For this review, take the finished solid that the model builds, in its own axes (mm). A direction names the side the tool comes from. Give positions to 0.01 mm unless a question says otherwise; leave off trailing zeros. Loops run counter-clockwise (first coordinate to the right, second up) from the corner with the lowest first, then second, coordinate; pieces in that order, holes last. Notation, with made-up numbers: (81.25, 73.25) - (140.25, 73.25) arc R14 cw to (140.25, 85.25) - close; hole circle Ø5 at (-27, -32). An arc over 180 degrees is marked (long way). Answer in a Markdown table with one row per item.
```python
from build123d import *

# Parameters (mm, degrees)
SKETCH_1_R          = 15.5
SKETCH_1_R_2        = 2
EXTRUDE_1_DEPTH     = 3
FILLET_1_R          = 3
SKETCH_5_R          = 15.5
SKETCH_5_R_2        = 2
EXTRUDE_3_DEPTH     = 2
EXTRUDE_5_DEPTH     = 7
FILLET_4_R          = 1
SKETCH_8_R          = 1.5
CUT_EXTRUDE_3_DEPTH = 35.179672449


with BuildPart() as part:
    # 草图1 → 凸台-拉伸1 (new body)
    with BuildSketch(Plane.XY):
        Circle(SKETCH_1_R)
        with Locations((-10.392304845, -6)):
            Circle(SKETCH_1_R_2, mode=Mode.SUBTRACT)
        with Locations((10.392304845, -6)):
            Circle(SKETCH_1_R_2, mode=Mode.SUBTRACT)
        with Locations((-10.392304845, 6)):
            Circle(SKETCH_1_R_2, mode=Mode.SUBTRACT)
        with BuildLine():
            ThreePointArc((2.604308084, 8.091203829), (5.825, 10.089195954), (5.705034021, 6.300998875))
            ThreePointArc((5.705034021, 6.300998875), (8.5, 0), (5.705034021, -6.300998875))
            ThreePointArc((5.705034021, -6.300998875), (5.825, -10.089195954), (2.604308084, -8.091203829))
            ThreePointArc((2.604308084, -8.091203829), (-4.25, -7.361215932), (-8.309342105, -1.790204954))
            ThreePointArc((-8.309342105, -1.790204954), (-11.65, 0), (-8.309342105, 1.790204954))
            ThreePointArc((-8.309342105, 1.790204954), (-4.25, 7.361215932), (2.604308084, 8.091203829))
        make_face(mode=Mode.SUBTRACT)
        with Locations((10.392304845, 6)):
            Circle(SKETCH_1_R_2, mode=Mode.SUBTRACT)
    extrude(amount=EXTRUDE_1_DEPTH)

    # 圆角1
    fillet_1_edges = [part.edges().sort_by_distance(p)[0] for p in [
        (-8.309342105, 1.790204954, 1.5),
        (-8.309342105, -1.790204954, 1.5),
        (2.604308084, -8.091203829, 1.5),
        (5.705034021, -6.300998875, 1.5),
        (5.705034021, 6.300998875, 1.5),
        (2.604308084, 8.091203829, 1.5),
    ]]
    fillet(fillet_1_edges, radius=FILLET_1_R)

    # 草图5 → 凸台-拉伸3 (add)
    with BuildSketch(Plane.XY.offset(3)):
        Circle(SKETCH_5_R)
        with Locations((-10.392304845, -6)):
            Circle(SKETCH_5_R_2, mode=Mode.SUBTRACT)
        with Locations((10.392304845, -6)):
            Circle(SKETCH_5_R_2, mode=Mode.SUBTRACT)
        with Locations((10.392304845, 6)):
            Circle(SKETCH_5_R_2, mode=Mode.SUBTRACT)
        with Locations((-10.392304845, 6)):
            Circle(SKETCH_5_R_2, mode=Mode.SUBTRACT)
    extrude(amount=EXTRUDE_3_DEPTH)

    # 草图7 → 凸台-拉伸5 (add)
    with BuildSketch(Plane.XY.offset(5)):
        with BuildLine():
            Line((9, 12.5), (-9, 12.5))
            Line((-9, 12.5), (-9, 9.481951639))
            ThreePointArc((-9, 9.481951639), (-7.287176573, 8.102540942), (-6.642304845, 6))
            ThreePointArc((-6.642304845, 6), (-7.287176573, 3.897459058), (-9, 2.518048361))
            Line((-9, 2.518048361), (-9, -2.518048361))
            ThreePointArc((-9, -2.518048361), (-7.287176573, -3.897459058), (-6.642304845, -6))
            ThreePointArc((-6.642304845, -6), (-7.287176573, -8.102540942), (-9, -9.481951639))
            Line((-9, -9.481951639), (-9, -12.5))
            Line((-9, -12.5), (9, -12.5))
            Line((9, -12.5), (9, -9.481951639))
            ThreePointArc((9, -9.481951639), (6.642304845, -6), (9, -2.518048361))
            Line((9, -2.518048361), (9, 2.518048361))
            ThreePointArc((9, 2.518048361), (6.642304845, 6), (9, 9.481951639))
            Line((9, 9.481951639), (9, 12.5))
        make_face()
    extrude(amount=EXTRUDE_5_DEPTH)

    # 圆角4
    fillet_4_edges = [part.edges().sort_by_distance(p)[0] for p in [
        (9, -9.481951639, 8.5),
        (9, -2.518048361, 8.5),
        (9, 2.518048361, 8.5),
        (9, 9.481951639, 8.5),
        (9, 12.5, 8.5),
        (-9, 12.5, 8.5),
        (-9, 9.481951639, 8.5),
        (-9, 2.518048361, 8.5),
        (-9, -2.518048361, 8.5),
        (-9, -9.481951639, 8.5),
        (-9, -12.5, 8.5),
        (9, -12.5, 8.5),
    ]]
    fillet(fillet_4_edges, radius=FILLET_4_R)

    # 草图8 → 切除-拉伸3 (cut, through all)
    with BuildSketch(Plane(origin=(0, 12.5, 0), x_dir=(1, 0, 0), z_dir=(0, 1, 0))):
        with Locations(Location((-4.75, -8.5, 0), (0, 0, 270))):
            Circle(SKETCH_8_R)
        with Locations(Location((4.75, -8.5, 0), (0, 0, 270))):
            Circle(SKETCH_8_R)
    extrude(amount=-CUT_EXTRUDE_3_DEPTH, mode=Mode.SUBTRACT)


solid = part.part
```
1. We need section A-A, the plane z = 8.5. Count the separate pieces of the cut face and the enclosed holes in it, and give its area (3 significant figures).
Values:
| item | result |
|---|---|
| separate pieces | 3 |
| enclosed holes | 0 |
| area | 251 mm^2 |
2. Clearance check with flat-ended pins moving along their axes: pin 1 (5.5 mm diameter, centred on x = 0, z = 8.5, fed in from -Y); pin 2 (5 mm diameter, centred on y = -7.5, z = 4, fed in from -X); pin 3 (2 mm diameter, centred on x = -3.5, z = 9.5, fed in from +Y). State where each tip first meets the part, or that it passes through.
Values:
| item | result |
|---|---|
| pin 1 | stops at y = -12.5 |
| pin 2 | stops at x = -14.67 |
| pin 3 | stops at y = 12.5 |
3. We need section B-B, the plane y = 0. Give the boundary of the cut face in (x, z), and give its area (3 significant figures).
Values:
| item | result |
|---|---|
| outline | (-15.5, 0) - (-11.65, 0) - (-11.65, 3) - (8.5, 3) - (8.5, 0) - (15.5, 0) - (15.5, 5) - (9, 5) - (9, 12) - (-9, 12) - (-9, 5) - (-15.5, 5) - close; hole circle Ø3 at (-4.75, 8.5); hole circle Ø3 at (4.75, 8.5) |
| area | 206 mm^2 |
4. Mouldability with a two-part tool opening along Y and no side actions: class faces 4 (the face through (8.699, -12.215, 8.549)), 5 (the face through (0, 0, 12)), 6 (the face through (8.394, 6.088, 2.465)) as released by +Y, released by -Y, zero draft, split by the parting line, or undercut.
Values:
| item | result |
|---|---|
| face 4 | released by -Y |
| face 5 | zero draft |
| face 6 | undercut |
5. We need section D-D, the plane x = 0. Give the boundary of the cut face in (y, z).
Values:
| item | result |
|---|---|
| outline | (-15.5, 0) - (-8.5, 0) - (-8.5, 3) - (8.5, 3) - (8.5, 0) - (15.5, 0) - (15.5, 5) - (12.5, 5) - (12.5, 12) - (-12.5, 12) - (-12.5, 5) - (-15.5, 5) - close |
6. We need section C-C, the plane x = -4.75. Give the boundary of the cut face in (y, z), and give its area (3 significant figures).
Values:
| item | result |
|---|---|
| outline | (-14.75, 0) - (-7.05, 0) - (-7.05, 3) - (7.05, 3) - (7.05, 0) - (14.75, 0) - (14.75, 5) - (12.5, 5) - (12.5, 7) - (-12.5, 7) - (-12.5, 5) - (-14.75, 5) - close; (-12.5, 10) - (12.5, 10) - (12.5, 12) - (-12.5, 12) - close |
| area | 205 mm^2 |
7. Wall thickness on line 1 (X direction, y = 11.5, z = 7.75); line 2 (Y direction, x = -8, z = 11.25); line 3 (Y direction, x = 7.5, z = 7.75): over which ranges is each line inside the solid? List them lowest first. Write a range as [from, to].
Values:
| item | result |
|---|---|
| line 1 | x = [-9, -6.05], [-3.45, 3.45], [6.05, 9] |
| line 2 | y = [-12.5, -8.89], [-3.11, 3.11], [8.89, 12.5] |
| line 3 | y = [-12.5, -8.39], [-3.61, 3.61], [8.39, 12.5] |
8. For faces 1 (the face through (-8.863, -9.599, 8.549)), 2 (the face through (5.79, 10.11, 1.48)), 3 (the face through (7, -6, 5)), list the 3-axis set-ups (+Z, -Z, +X, -X, +Y, -Y) from which the entire face can be reached by the end or side of a thin tool; tool diameter is ignored.
Values:
| item | result |
|---|---|
| face 1 | +Z, -X |
| face 2 | -Z |
| face 3 | +Z |
